The listing builds one solid part. Answer for the finished solid, in the listing's coordinates (mm). Coordinates: 2 decimals unless noted, no trailing zeros. Write each loop counter-clockwise with the first axis right and the second up, starting at its lowest first coordinate (ties: lowest second). Pieces come first, ordered by that corner, then holes.
(1) For a pull along Z with two mould halves and no side action, classify faces 1 (the cylindrical face through (-56.809, -32.023, 106.239)), 2 (the flat face through (-33.98, -102.99, 40.22)), 3 (the cylindrical face through (-69.891, -6.983, 25.88)), 4 (the cylindrical face through (-31.495, -125.628, -28.995)) as +Z half, -Z half, draft (parallel to the pull), parting line (faces both ways), or undercut.
(2) The part is cut by section A-A on y = -144.5. Determine the outline of the cut face in (x, z).
(3) The part is cut by section B-B on y = -67. Determine the outline of the cut face in (x, z).
(4) Straight lines are drawn through the part: line 1 (X direction, y = -98, z = -8); line 2 (X direction, y = -39.5, z = 29.5). For each, find the intervals that lie inside material, in ascending order.
from build123d import *

# Parameters (mm, degrees)
BOSS_EXTRUDE1_DEPTH                               = 3.175
F_6_CLEARANCE_HOLE2_D                             = 4.3053
CUT_EXTRUDE1_DEPTH                                = 75.708255191
CUT_EXTRUDE11_DEPTH                               = 75.708255191
SKETCH112_R                                       = 6.35
CUT_EXTRUDE13_DEPTH                               = 75.708255191
CSK_FOR_6_FLAT_HEAD_MACHINE_SCREW_100_D           = 4.3053
CSK_FOR_6_FLAT_HEAD_MACHINE_SCREW_100_CSINK_D     = 7.0866
CSK_FOR_6_FLAT_HEAD_MACHINE_SCREW_100_CSINK_ANGLE = 100
F_2_CLEARANCE_HOLE1_D                             = 2.2606
F_2_CLEARANCE_HOLE1_DEPTH                         = 3.175


with BuildPart() as part:
    # Sketch2 → Boss-Extrude1 (new body)
    with BuildSketch(Plane(origin=(-64.088304417, -22.345630777, 3.470722632), x_dir=(-0.153926818, 0.29499983, -0.943017304), z_dir=(0.943017304, 0.328801279, -0.051069404))):
        with BuildLine():
            Line((-121.846755419, -165.728170273), (-69.459255419, -165.728170273))
            ThreePointArc((-69.459255419, -165.728170273), (-68.336723403, -165.263202289), (-67.871755419, -164.140670273))
            Line((-67.871755419, -164.140670273), (-67.871755419, -120.325670273))
            ThreePointArc((-67.871755419, -120.325670273), (-67.406787434, -119.203138258), (-66.284255419, -118.738170273))
            Line((-66.284255419, -118.738170273), (-3.736755419, -118.738170273))
            ThreePointArc((-3.736755419, -118.738170273), (3.883244581, -111.118170273), (-3.736755419, -103.498170273))
            Line((-3.736755419, -103.498170273), (-10.721755419, -103.498170273))
            ThreePointArc((-10.721755419, -103.498170273), (-12.966819449, -102.568234304), (-13.896755419, -100.323170273))
            Line((-13.896755419, -100.323170273), (-13.896755419, 18.421829727))
            ThreePointArc((-13.896755419, 18.421829727), (-15.756627358, 22.911957787), (-20.246755419, 24.771829727))
            Line((-20.246755419, 24.771829727), (-96.446755419, 24.771829727))
            ThreePointArc((-96.446755419, 24.771829727), (-100.936883479, 22.911957787), (-102.796755419, 18.421829727))
            Line((-102.796755419, 18.421829727), (-102.796755419, -30.790670273))
            ThreePointArc((-102.796755419, -30.790670273), (-103.261723403, -31.913202289), (-104.384255419, -32.378170273))
            Line((-104.384255419, -32.378170273), (-121.846755419, -32.378170273))
            ThreePointArc((-121.846755419, -32.378170273), (-126.336883479, -34.238042213), (-128.196755419, -38.728170273))
            Line((-128.196755419, -38.728170273), (-128.196755419, -159.378170273))
            ThreePointArc((-128.196755419, -159.378170273), (-126.336883479, -163.868298334), (-121.846755419, -165.728170273))
        make_face()
    extrude(amount=-BOSS_EXTRUDE1_DEPTH)

    # #6 Clearance Hole2 (through all)
    with Locations(Plane(origin=(-67.082384355, -23.389574839, 3.632867989), x_dir=(0.048222256, 0.016813625, 0.998695107), z_dir=(-0.943017304, -0.328801279, 0.051069404))):
        with Locations((94.496598047, -13.438577508), (27.821256, 9.809074133), (102.303221602, -76.684769209), (58.183274109, -19.607002634), (18.688641338, -122.850003783), (-33.055104908, -106.153526298), (79.375410017, -137.620951141), (62.581514662, -190.608465154)):
            Hole(F_6_CLEARANCE_HOLE2_D / 2)

    # Sketch11 → Cut-Extrude1 (cut, through all)
    with BuildSketch(Plane(origin=(-30.199339451, -118.769533988, 70.606372837), x_dir=(0.153926818, -0.29499983, 0.943017304), z_dir=(-0.943017304, -0.328801279, 0.051069404))):
        with BuildLine():
            Line((-5.443361979, 7.786170805), (1.218801886, 7.786170805))
            ThreePointArc((1.218801886, 7.786170805), (-2.112280046, -3.415229195), (-5.443361979, 7.786170805))
        make_face()
    extrude(amount=-CUT_EXTRUDE1_DEPTH, mode=Mode.SUBTRACT)

    # Sketch111 → Cut-Extrude11 (cut, through all)
    with BuildSketch(Plane(origin=(-50.471339887, -59.482551247, 77.984343899), x_dir=(0.153926818, -0.29499983, 0.943017304), z_dir=(-0.943017304, -0.328801279, 0.051069404))):
        with BuildLine():
            Line((-5.443361979, 7.786170805), (1.218801886, 7.786170805))
            ThreePointArc((1.218801886, 7.786170805), (-2.112280046, -3.415229195), (-5.443361979, 7.786170805))
        make_face()
    extrude(amount=-CUT_EXTRUDE11_DEPTH, mode=Mode.SUBTRACT)

    # Sketch112 → Cut-Extrude13 (cut, through all)
    with BuildSketch(Plane(origin=(-67.082384355, -23.389574839, 3.632867989), x_dir=(0.048222256, 0.016813625, 0.998695107), z_dir=(-0.943017304, -0.328801279, 0.051069404))):
        with Locations((1.528822601, -97.230139831)):
            Circle(SKETCH112_R)
        Polygon((51.631528484, -170.516238748), (32.684219053, -163.909891699), (39.290566102, -144.962582268), (58.237875533, -151.568929317), align=None)
    extrude(amount=-CUT_EXTRUDE13_DEPTH, mode=Mode.SUBTRACT)

    # CSK for #6 Flat Head Machine Screw (100)1 (through all)
    with Locations(Plane(origin=(-67.082384355, -23.389574839, 3.632867989), x_dir=(0.048222256, 0.016813625, 0.998695107), z_dir=(-0.943017304, -0.328801279, 0.051069404))):
        with Locations((18.106841092, -36.568198954), (45.444415988, -93.174400017)):
            CounterSinkHole(CSK_FOR_6_FLAT_HEAD_MACHINE_SCREW_100_D / 2, CSK_FOR_6_FLAT_HEAD_MACHINE_SCREW_100_CSINK_D / 2, counter_sink_angle=CSK_FOR_6_FLAT_HEAD_MACHINE_SCREW_100_CSINK_ANGLE)

    # #2 Clearance Hole1
    with Locations(Plane(origin=(-64.088304417, -22.345630777, 3.470722632), x_dir=(-0.048222256, -0.016813625, -0.998695107), z_dir=(0.943017304, 0.328801279, -0.051069404))):
        with Locations((-34.795660006, -166.629937328), (-56.12643458, -148.848883687)):
            Hole(F_2_CLEARANCE_HOLE1_D / 2, depth=F_2_CLEARANCE_HOLE1_DEPTH)


solid = part.part
Model answer:
1. face 1: +Z half
1. face 2: -Z half
1. face 3: parting line
1. face 4: undercut
2. outline: (-24.44, 11.22) - (-20.91, 14.39) - (-16.62, 93.45) - (-19.96, 94) - close
3. outline: (-51.95, 2.26) - (-48.61, 1.71) - (-43.55, 95.16) - (-46.89, 95.7) - close
4. line 1: x = -41.7 to -38.33
4. line 2: x = -60.06 to -56.7
